Verification items for the finished model (mm, model axes). Round coordinates to 2 decimals unless told otherwise and drop trailing zeros. Write each loop counter-clockwise with the first axis right and the second up, starting at its lowest first coordinate (ties: lowest second). Pieces come first, ordered by that corner, then holes. Notation, with made-up numbers: M 8.25,49 L 45.25,49 A11 ccw 45.25,66 Z; hole C -6.75,73.25 d7. An arc over 180 degrees is marked long. One line per question, with ' | ' between items.
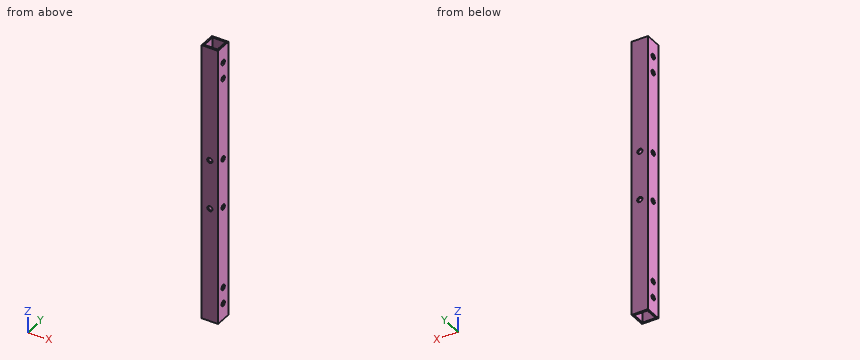
from build123d import *

# Parameters (mm, degrees)
SKETCH1_W           = 10
SKETCH1_H           = 10
SKETCH1_W_2         = 8
SKETCH1_H_2         = 8
BOSS_EXTRUDE1_DEPTH = 170
CUT_EXTRUDE1_REACH  = 172.367
SKETCH2_R           = 1.6
SKETCH3_R           = 1.6
CUT_EXTRUDE2_DEPTH  = 10


with BuildPart() as part:
    # Sketch1 → Boss-Extrude1 (new body)
    with BuildSketch(Plane.XY):
        Rectangle(SKETCH1_W, SKETCH1_H)
        Rectangle(SKETCH1_W_2, SKETCH1_H_2, mode=Mode.SUBTRACT)
    extrude(amount=BOSS_EXTRUDE1_DEPTH)

    # Cut-Extrude1: up to this face of the body (flat: up to its plane)
    cut_extrude1_end = Plane(part.part.faces().sort_by_distance((-5, 0, 85))[0])
    # Sketch2 → Cut-Extrude1 (cut, up to the picked face)
    with BuildSketch(Plane(origin=(5, 0, 0), x_dir=(0, 0, -1), z_dir=(1, 0, 0)), mode=Mode.PRIVATE) as cut_extrude1_sk1:
        with Locations(Location((-20, 0, 0), (0, 0, 90))):
            Circle(SKETCH2_R)
    cut_extrude1_tool1 = split(extrude(cut_extrude1_sk1.sketch, amount=-CUT_EXTRUDE1_REACH, mode=Mode.PRIVATE), bisect_by=cut_extrude1_end, keep=Keep.BOTH, mode=Mode.PRIVATE)
    # Sketch2 → Cut-Extrude1 (cut, up to the picked face)
    with BuildSketch(Plane(origin=(5, 0, 0), x_dir=(0, 0, -1), z_dir=(1, 0, 0)), mode=Mode.PRIVATE) as cut_extrude1_sk2:
        with Locations(Location((-10, 0, 0), (0, 0, 90))):
            Circle(SKETCH2_R)
    cut_extrude1_tool2 = split(extrude(cut_extrude1_sk2.sketch, amount=-CUT_EXTRUDE1_REACH, mode=Mode.PRIVATE), bisect_by=cut_extrude1_end, keep=Keep.BOTH, mode=Mode.PRIVATE)
    # Sketch2 → Cut-Extrude1 (cut, up to the picked face)
    with BuildSketch(Plane(origin=(5, 0, 0), x_dir=(0, 0, -1), z_dir=(1, 0, 0)), mode=Mode.PRIVATE) as cut_extrude1_sk3:
        with Locations(Location((-160, 0, 0), (0, 0, 90))):
            Circle(SKETCH2_R)
    cut_extrude1_tool3 = split(extrude(cut_extrude1_sk3.sketch, amount=-CUT_EXTRUDE1_REACH, mode=Mode.PRIVATE), bisect_by=cut_extrude1_end, keep=Keep.BOTH, mode=Mode.PRIVATE)
    # Sketch2 → Cut-Extrude1 (cut, up to the picked face)
    with BuildSketch(Plane(origin=(5, 0, 0), x_dir=(0, 0, -1), z_dir=(1, 0, 0)), mode=Mode.PRIVATE) as cut_extrude1_sk4:
        with Locations(Location((-150, 0, 0), (0, 0, 90))):
            Circle(SKETCH2_R)
    cut_extrude1_tool4 = split(extrude(cut_extrude1_sk4.sketch, amount=-CUT_EXTRUDE1_REACH, mode=Mode.PRIVATE), bisect_by=cut_extrude1_end, keep=Keep.BOTH, mode=Mode.PRIVATE)
    # Sketch2 → Cut-Extrude1 (cut, up to the picked face)
    with BuildSketch(Plane(origin=(5, 0, 0), x_dir=(0, 0, -1), z_dir=(1, 0, 0)), mode=Mode.PRIVATE) as cut_extrude1_sk5:
        with Locations(Location((-70, 0, 0), (0, 0, 90))):
            Circle(SKETCH2_R)
    cut_extrude1_tool5 = split(extrude(cut_extrude1_sk5.sketch, amount=-CUT_EXTRUDE1_REACH, mode=Mode.PRIVATE), bisect_by=cut_extrude1_end, keep=Keep.BOTH, mode=Mode.PRIVATE)
    # Sketch2 → Cut-Extrude1 (cut, up to the picked face)
    with BuildSketch(Plane(origin=(5, 0, 0), x_dir=(0, 0, -1), z_dir=(1, 0, 0)), mode=Mode.PRIVATE) as cut_extrude1_sk6:
        with Locations(Location((-100, 0, 0), (0, 0, 90))):
            Circle(SKETCH2_R)
    cut_extrude1_tool6 = split(extrude(cut_extrude1_sk6.sketch, amount=-CUT_EXTRUDE1_REACH, mode=Mode.PRIVATE), bisect_by=cut_extrude1_end, keep=Keep.BOTH, mode=Mode.PRIVATE)
    add(cut_extrude1_tool1.solids().sort_by(Axis((5, 0, 20), (-1, 0, 0)))[0], mode=Mode.SUBTRACT)
    add(cut_extrude1_tool2.solids().sort_by(Axis((5, 0, 10), (-1, 0, 0)))[0], mode=Mode.SUBTRACT)
    add(cut_extrude1_tool3.solids().sort_by(Axis((5, 0, 160), (-1, 0, 0)))[0], mode=Mode.SUBTRACT)
    add(cut_extrude1_tool4.solids().sort_by(Axis((5, 0, 150), (-1, 0, 0)))[0], mode=Mode.SUBTRACT)
    add(cut_extrude1_tool5.solids().sort_by(Axis((5, 0, 70), (-1, 0, 0)))[0], mode=Mode.SUBTRACT)
    add(cut_extrude1_tool6.solids().sort_by(Axis((5, 0, 100), (-1, 0, 0)))[0], mode=Mode.SUBTRACT)

    # Sketch3 → Cut-Extrude2 (cut)
    with BuildSketch(Plane(origin=(0, 5, 0), x_dir=(1, 0, 0), z_dir=(0, 1, 0))):
        with Locations(Location((0, -70, 0), (0, 0, 270))):
            Circle(SKETCH3_R)
        with Locations(Location((0, -100, 0), (0, 0, 270))):
            Circle(SKETCH3_R)
    extrude(amount=-CUT_EXTRUDE2_DEPTH, mode=Mode.SUBTRACT)


solid = part.part
1. Section check B-B, the plane z = 70. Record the cut outline in (x, y).
Results:
outline: M -5,-5 L -1.6,-5 L -1.6,-4 L -4,-4 L -4,-1.6 L -5,-1.6 Z; M -5,1.6 L -4,1.6 L -4,4 L -1.6,4 L -1.6,5 L -5,5 Z; M 1.6,-5 L 5,-5 L 5,-1.6 L 4,-1.6 L 4,-4 L 1.6,-4 Z; M 1.6,4 L 4,4 L 4,1.6 L 5,1.6 L 5,5 L 1.6,5 Z
2. Thickness scan on line 1 (X direction, y = -2, z = 56); line 2 (Y direction, x = 4.6, z = 70). Record the ranges inside material, lowest first.
Results:
line 1: x = -5 to -4, 4 to 5 | line 2: y = -5 to -1.6, 1.6 to 5
3. Section check C-C, the plane z = 156.5. Record the cut outline in (x, y), then the cut area to 3 significant figures.
Results:
outline: M -5,-5 L 5,-5 L 5,5 L -5,5 Z; hole M -4,-4 L 4,-4 L 4,4 L -4,4 Z | area: 36.0 mm2
4. Section check A-A, the plane z = 20. Record the cut outline in (x, y).
Results:
outline: M -5,-5 L 5,-5 L 5,-1.6 L 4,-1.6 L 4,-4 L -4,-4 L -4,-1.6 L -5,-1.6 Z; M -5,1.6 L -4,1.6 L -4,4 L 4,4 L 4,1.6 L 5,1.6 L 5,5 L -5,5 Z
